Build history of the part. All positions in model axes, mm. A direction names the side the tool comes from. Give positions to 0.01 mm unless a question says otherwise; leave off trailing zeros. Order: outer loops, then holes, each group sorted by start corner. A loop starts at its lowest first (then second) coordinate and runs counter-clockwise, first axis right, second up. Notation, with made-up numbers: (36, 18) -> (85, 18) arc R23 cw to (85, 54) -> close; hole circle Ø4 at (47, -29.5). An arc over 180 degrees is marked (long way). One line per item, written item: value. Start each with the question number.
(1) Which spindle directions (+Z, -Z, +X, -X, +Y, -Y) get a long thin tool onto all of the face, cutting with end or side? Do faces 1 (the cylindrical face through (9.175, 29.114, 3.451)), 2 (the flat face through (12, 2, 1)), 3 (the flat face through (-12, 2, 1)), 4 (the cylindrical face through (-20.587, 17.633, -0.74)). Say none if no direction does.
(2) Two-plate mould, pull along Y, no slides. Class faces 5 (the cylindrical face through (-20.11, 17.84, 0.47)), 6 (the flat face through (-22, 4.6, 1)), 7 (the cylindrical face through (10.746, 30.045, 4.719)), 8 (the flat face through (11, 26, 7)): +Y half, -Y half, draft (parallel to the pull), parting line (faces both ways), or undercut.
(3) Saw through at D-D on x = 1.5. Give the cut face in (y, z), plus the area to 3 significant figures.
(4) Pin check, flat tips, straight feed: pin 1 (6 mm diameter, centred on x = -20, y = 40.2, fed in from -Z); pin 2 (1.2 mm diameter, centred on x = -18, z = 1.5, fed in from -Y); pin 3 (3 mm diameter, centred on y = 2.5, z = 2, fed in from -X); pin 4 (19 mm diameter, centred on x = 13.5, y = 30.5, fed in from +Z). Stop position of each tip, or through.
(5) Saw through at A-A on y = 18.85. Give the cut face in (x, z).
(6) Saw through at B-B on z = 1.5. Give the cut face in (x, y).
(7) Saw through at C-C on y = 27.65. Give the cut face in (x, z).
(8) Probe line 1 (X direction, y = 27.5, z = 3.5); line 2 (Y direction, x = -1.5, z = -0.35); line 3 (Y direction, x = -20, z = 0.9). List the from-to ranges inside material, lowest first.
Autodesk Inventor part; units mm, degrees
ref_plane "YZ Plane" through (0, 0, 0) normal (1, 0, 0) x (0, 1, 0)
ref_plane "XZ Plane" through (0, 0, 0) normal (0, 1, 0) x (-1, 0, 0)
ref_plane "XY Plane" through (0, 0, 0) normal (0, 0, 1) x (1, 0, 0)
sketch "Sketch1" plane through (0, 0, 0) normal (0, 0, 1) x (1, 0, 0)
  circle A0 centre (0, 0) radius 3.6
  line L0 (32, 4.6) -> (12, 4.6)
  line L1 (-32, 4.6) -> (-32, 40.1)
  line L2 (-20, 52.1) -> (20, 52.1)
  line L3 (32, 40.1) -> (32, 4.6)
  circle A1 centre (-19, 18.85) radius 2
  circle A2 centre (-1.5, 37.75) radius 2
  circle A3 centre (9.5, 27.65) radius 1.5
  circle A4 centre (23.5, 27.65) radius 1.5
  circle A5 centre (9.5, 27.65) radius 2.7
  circle A6 centre (23.5, 27.65) radius 2.7
  circle A7 centre (-20, 40.2) radius 2.5
  circle A8 centre (-19, 18.85) radius 1.5
  circle A9 centre (-1.5, 37.75) radius 1.5
  circle A10 centre (20, 40.2) radius 2.5
  arc A11 (-20, 52.1) -> (-32, 40.1) centre (-20, 40.1) ccw
  arc A12 (32, 40.1) -> (20, 52.1) centre (20, 40.1) ccw
  arc A13 (-12, 0) -> (12, 0) centre (0, 0) ccw
  line L4 (-12, 0) -> (-12, 4.6)
  line L5 (12, 4.6) -> (12, 0)
  line L6 (-12, 4.6) -> (-32, 4.6)
  point P0 (-32, 52.1)
  dimension "d0" = 7.2
  dimension "d1" = 52.1
  dimension "d2" = 4.6
  dimension "d3" = 32
  dimension "d4" = 32
  dimension "d5" = 4
  dimension "d6" = 33.25
  dimension "d7" = 19
  dimension "d8" = 4
  dimension "d9" = 1.5
  dimension "d10" = 14.35
  dimension "d11" = 3
  dimension "d12" = 9.5
  dimension "d13" = 24.45
  dimension "d14" = 3
  dimension "d15" = 23.5
  dimension "d16" = 1.2
  dimension "d17" = 1.2
  dimension "d18" = 20
  dimension "d19" = 11.9
  dimension "d20" = 5
  dimension "d21" = 3
  dimension "d22" = 3
  dimension "d23" = 5
  dimension "d24" = 20
  dimension "d25" = 12
  dimension "d27" = 12
extrude "Extrusion1" add sketch "Sketch1" along normal blind 2.5 contours L0 L5 A13 L4 L6 L1 A11 L2 A12 L3
extrude "Extrusion2" add sketch "Sketch1" along normal blind 7 contours A5 | A6
extrude "Extrusion3" add sketch "Sketch1" along normal blind 2.5 and the other way blind 1.5 contours A1 | A2
properties part number "ENDER 3 E_PLATE" material "Steel, High Strength, Low Alloy"
Results below:
1. face 1: +Z, -Z
1. face 2: +Z, -Z, +X, -Y
1. face 3: +Z, -Z, -X, -Y
1. face 4: -Z
2. face 5: undercut
2. face 6: -Y half
2. face 7: parting line
2. face 8: draft
3. outline: (-11.91, 0) -> (-3.27, 0) -> (-3.27, 2.5) -> (-11.91, 2.5) -> close; (3.27, 0) -> (52.1, 0) -> (52.1, 2.5) -> (3.27, 2.5) -> close
3. area: 144 mm²
4. pin 1: stops at z = 0
4. pin 2: stops at y = 4.6
4. pin 3: stops at x = -12
4. pin 4: stops at z = 7
5. outline: (-32, 0) -> (-21, 0) -> (-21, -1.5) -> (-20.5, -1.5) -> (-20.5, 2.5) -> (-32, 2.5) -> close; (-17.5, -1.5) -> (-17, -1.5) -> (-17, 0) -> (32, 0) -> (32, 2.5) -> (-17.5, 2.5) -> close
6. outline: (-32, 4.6) -> (-12, 4.6) -> (-12, 0) arc R12 ccw to (12, 0) -> (12, 4.6) -> (32, 4.6) -> (32, 40.1) arc R12 ccw to (20, 52.1) -> (-20, 52.1) arc R12 ccw to (-32, 40.1) -> close; hole circle Ø5 at (-20, 40.2); hole circle Ø3 at (-19, 18.85); hole circle Ø7.2 at (0, 0); hole circle Ø3 at (-1.5, 37.75); hole circle Ø3 at (9.5, 27.65); hole circle Ø5 at (20, 40.2); hole circle Ø3 at (23.5, 27.65)
7. outline: (-32, 0) -> (8, 0) -> (8, 7) -> (6.8, 7) -> (6.8, 2.5) -> (-32, 2.5) -> close; (11, 0) -> (22, 0) -> (22, 7) -> (20.8, 7) -> (20.8, 2.5) -> (12.2, 2.5) -> (12.2, 7) -> (11, 7) -> close; (25, 0) -> (32, 0) -> (32, 2.5) -> (26.2, 2.5) -> (26.2, 7) -> (25, 7) -> close
8. line 1: x = 6.8 to 8.01, 10.99 to 12.2, 20.8 to 22.01, 24.99 to 26.2
8. line 2: y = 35.75 to 36.25, 39.25 to 39.75
8. line 3: y = 4.6 to 17.73, 19.97 to 37.7, 42.7 to 52.1
